Check sheet for the drawn part. Datum: minimum x, y, z corner. Units: mm. A direction names the side the tool comes from. Give positions to 0.01 mm unless a question says otherwise; leave off trailing zeros. Order: outer loops, then holes, each group sorted by start corner. A loop starts at its lowest first (then second) coordinate and runs counter-clockwise, first axis right, second up. Notation, with made-up numbers: M 17,26.5 L 38,26.5 A29 ccw 38,62.5 Z; hole C -6,79.25 d9. An arc over 180 degrees is marked long. Put each result on its own line as item: value. Start each with the question number.
Q1. Section check A-A on y = 10. Record the cut outline in (x, z).
Q2. Access from +Z, -Z, +X, -X, +Y, -Y to the whole of each face (thin tool, end or side, straight path). Record for the marked faces 1 and 2.
Q3. Material ranges on L1, parallel to X at y = 10, z = 2.35; L2, parallel to Z at x = 6, y = 6.75; L3, parallel to Y at x = 40, z = 15, recorded low to high.
Q4. Section check D-D on z = 2.25. Record the cut outline in (x, y).
Q5. Section check B-B on x = 10. Record the cut outline in (y, z).
Q6. Section check C-C on x = 20. Record the cut outline in (y, z).
Q7. Go/stop test with flat-tipped pins: pin 1 (13.5 mm diameter, centred on x = 54, z = 13, fed in from -Y); pin 2 (8.5 mm diameter, centred on x = 60, y = 11.5, fed in from +Z); pin 3 (6 mm diameter, centred on x = 16.5, z = 6.5, fed in from -Y). Record where each tip stops, or that it passes through.
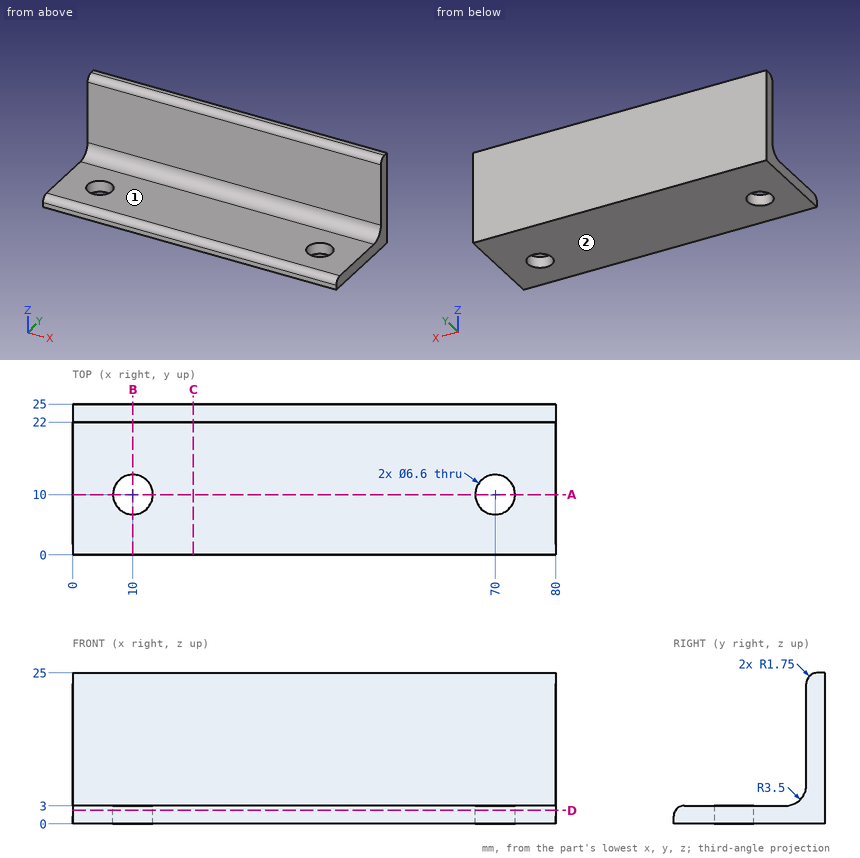
Results found:
1. outline: M 0,0 L 6.7,0 L 6.7,3 L 0,3 Z; M 13.3,0 L 66.7,0 L 66.7,3 L 13.3,3 Z; M 73.3,0 L 80,0 L 80,3 L 73.3,3 Z
2. face 1: +Z, +X, -X, -Y
2. face 2: -Z, +X, -X, +Y, -Y
3. L1: x = 0 to 6.7, 13.3 to 66.7, 73.3 to 80
3. L2: z = 0 to 3
3. L3: y = 22 to 25
4. outline: M 0,0.31 L 80,0.31 L 80,25 L 0,25 Z; hole C 10,10 d6.6; hole C 70,10 d6.6
5. outline: M 0,0 L 6.7,0 L 6.7,3 L 1.75,3 A1.75 ccw 0,1.25 Z; M 13.3,0 L 25,0 L 25,25 L 23.75,25 A1.75 ccw 22,23.25 L 22,6.5 A3.5 cw 18.5,3 L 13.3,3 Z
6. outline: M 0,0 L 25,0 L 25,25 L 23.75,25 A1.75 ccw 22,23.25 L 22,6.5 A3.5 cw 18.5,3 L 1.75,3 A1.75 ccw 0,1.25 Z
7. pin 1: stops at y = 21.99
7. pin 2: stops at z = 3
7. pin 3: stops at y = 20.3
